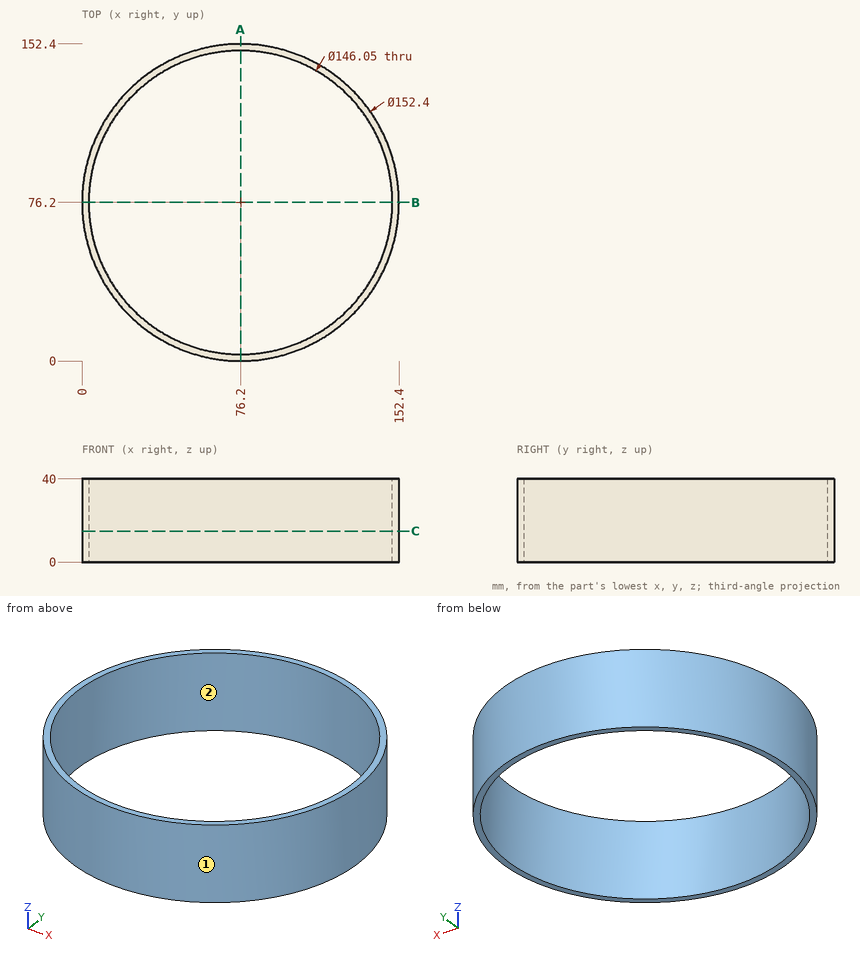
Answer from the drawing. Dimensions are ordinates in mm from the lowest x, y and z of the part. Coordinates: 2 decimals unless noted, no trailing zeros. Loops run counter-clockwise (first coordinate to the right, second up) from the corner with the lowest first, then second, coordinate; pieces in that order, holes last.
1) Consider probe 1 along Y at (x, z) = (76.2, 21) (3 decimals); probe 2 along X at (y, z) = (30, 34.5); probe 3 along X at (y, z) = (104.5, 30). Determine where each line is inside the solid, lowest interval first.
Results:
probe 1: y = 0 to 3.175, 149.225 to 152.4
probe 2: x = 15.6 to 19.65, 132.75 to 136.8
probe 3: x = 5.45 to 8.88, 143.52 to 146.95
2) Flat-ended cylindrical pins translate along their axes: pin 1 (5 mm diameter, centred on y = 49, z = 21, fed in from -X); pin 2 (5 mm diameter, centred on y = 41, z = 15, fed in from +X); pin 3 (5 mm diameter, centred on y = 110, z = 11, fed in from +X). Find the tip coordinate at first contact, or state that the pin passes through.
Results:
pin 1: stops at x = 4.11
pin 2: stops at x = 145.03
pin 3: stops at x = 145.67
3) Section C-C (z = 15) is taken. Give the vertices of the cut face in (x, y) (3 decimals).
Results:
outline: circle Ø152.4 at (76.2, 76.2); hole circle Ø146.05 at (76.2, 76.2)
4) Section A-A (x = 76.2) is taken. Give the vertices of the cut face in (y, z) (3 decimals).
Results:
outline: (0, 0) - (3.175, 0) - (3.175, 40) - (0, 40) - close; (149.225, 0) - (152.4, 0) - (152.4, 40) - (149.225, 40) - close
5) For a pull along X with two mould halves and no side action, classify the marked faces 1 and 2 as +X half, -X half, draft (parallel to the pull), parting line (faces both ways), or undercut.
Results:
face 1: parting line
face 2: undercut
